from build123d import *

# Parameters (mm, degrees)
SKETCH1_R              = 56.531668112
BOSS_EXTRUDE1_DEPTH    = 5
CUT_EXTRUDE1_START     = -9.696123263
CUT_EXTRUDE1_OUTLINE_R = 56.531668112
CUT_EXTRUDE1_DEPTH     = 5
CUT_EXTRUDE2_DEPTH     = 93.989824492


# Read off the part's stored shape, not the designer's step: Cut-Extrude1
with BuildPart() as part:
    # Sketch1 → Boss-Extrude1 (new body)
    with BuildSketch(Plane(origin=(0, 0, 0), x_dir=(1, 0, 0), z_dir=(0, 1, 0))):
        with Locations(Location((0, 0, 0), (0, 0, 270))):
            Circle(SKETCH1_R)
    extrude(amount=BOSS_EXTRUDE1_DEPTH)

    # Cut-Extrude1 outline → Cut-Extrude1 (cut)
    with BuildSketch(Plane(origin=(0.053951493, 9.696123263, -2.690451675), x_dir=(0, 0, 1), z_dir=(0, 1, 0)).offset(CUT_EXTRUDE1_START)):
        with Locations((2.690451675, -0.053951493)):
            Circle(CUT_EXTRUDE1_OUTLINE_R)
        with BuildLine():
            ThreePointArc((-0.274694701, 5.590628471), (0.097098839, 5.770814345), (0.479781475, 5.926542907))
            ThreePointArc((0.479781475, 5.926542907), (0.311357577, 7.137787092), (0.620358822, 8.321001915))
            ThreePointArc((0.620358822, 8.321001915), (0.896797518, 8.384527858), (1.175175163, 8.438931768))
            ThreePointArc((1.175175163, 8.438931768), (1.938718671, 7.48369337), (2.277513178, 6.308662576))
            ThreePointArc((2.277513178, 6.308662576), (2.690451674, 6.322048507), (3.103390171, 6.308662576))
            ThreePointArc((3.103390171, 6.308662576), (3.442184678, 7.483693371), (4.205728187, 8.438931768))
            ThreePointArc((4.205728187, 8.438931768), (4.484105832, 8.384527858), (4.760544528, 8.321001915))
            ThreePointArc((4.760544528, 8.321001915), (5.069545773, 7.137787092), (4.901121875, 5.926542907))
            ThreePointArc((4.901121875, 5.926542907), (5.283804511, 5.770814345), (5.65559805, 5.590628471))
            ThreePointArc((5.65559805, 5.590628471), (6.443030314, 6.526272375), (7.529092477, 7.088364951))
            ThreePointArc((7.529092477, 7.088364951), (7.761275046, 6.925438117), (7.987976033, 6.754966533))
            ThreePointArc((7.987976033, 6.754966533), (7.789005891, 5.548363877), (7.142485611, 4.510341424))
            ThreePointArc((7.142485611, 4.510341424), (7.428743082, 4.212425253), (7.695105184, 3.89659521))
            ThreePointArc((7.695105184, 3.89659521), (8.795021012, 4.431070894), (10.015811815, 4.502826734))
            ThreePointArc((10.015811815, 4.502826734), (10.161652833, 4.259548507), (10.299417449, 4.011607367))
            ThreePointArc((10.299417449, 4.011607367), (9.626879667, 2.990249439), (8.614052233, 2.304932231))
            ThreePointArc((8.614052233, 2.304932231), (8.754388023, 1.916340863), (8.869262259, 1.519476535))
            ThreePointArc((8.869262259, 1.519476535), (10.091476213, 1.560368296), (11.235909836, 1.129380165))
            ThreePointArc((11.235909836, 1.129380165), (11.270192066, 0.84781556), (11.295199558, 0.56527614))
            ThreePointArc((11.295199558, 0.56527614), (10.265382027, -0.094234996), (9.061374505, -0.308349388))
            ThreePointArc((9.061374505, -0.308349388), (9.03152328, -0.720424975), (8.975046852, -1.12970214))
            ThreePointArc((8.975046852, -1.12970214), (10.108227036, -1.589464859), (10.978420508, -2.448675198))
            ThreePointArc((10.978420508, -2.448675198), (10.895216241, -2.719841103), (10.803142587, -2.98812517))
            ThreePointArc((10.803142587, -2.98812517), (9.594110114, -3.171754047), (8.407106342, -2.8776433))
            ThreePointArc((8.407106342, -2.8776433), (8.212229649, -3.241951493), (7.994167845, -3.592873756))
            ThreePointArc((7.994167845, -3.592873756), (8.84237711, -4.473793803), (9.287866075, -5.612661077))
            ThreePointArc((9.287866075, -5.612661077), (9.101562084, -5.826541234), (8.908327655, -6.034181196))
            ThreePointArc((8.908327655, -6.034181196), (7.729132938, -5.710176712), (6.764376652, -4.958695246))
            ThreePointArc((6.764376652, -4.958695246), (6.438170443, -5.212243849), (6.09622813, -5.444133562))
            ThreePointArc((6.09622813, -5.444133562), (6.512803388, -6.593891859), (6.456558756, -7.81549557))
            ThreePointArc((6.456558756, -7.81549557), (6.199368695, -7.935108156), (5.938385479, -8.046201177))
            ThreePointArc((5.938385479, -8.046201177), (4.992921997, -7.270586652), (4.417228324, -6.191672439))
            ThreePointArc((4.417228324, -6.191672439), (4.016096616, -6.290620595), (3.609398725, -6.363381921))
            ThreePointArc((3.609398725, -6.363381921), (3.52231033, -7.583174812), (2.974057309, -8.67628858))
            ThreePointArc((2.974057309, -8.67628858), (2.690451675, -8.680951493), (2.406846041, -8.67628858))
            ThreePointArc((2.406846041, -8.67628858), (1.85859302, -7.583174812), (1.771504625, -6.363381921))
            ThreePointArc((1.771504625, -6.363381921), (1.364806734, -6.290620595), (0.963675026, -6.191672439))
            ThreePointArc((0.963675026, -6.191672439), (0.387981353, -7.270586652), (-0.557482129, -8.046201177))
            ThreePointArc((-0.557482129, -8.046201177), (-0.818465345, -7.935108156), (-1.075655406, -7.81549557))
            ThreePointArc((-1.075655406, -7.81549557), (-1.131900038, -6.593891859), (-0.71532478, -5.444133562))
            ThreePointArc((-0.71532478, -5.444133562), (-1.057267094, -5.212243849), (-1.383473303, -4.958695246))
            ThreePointArc((-1.383473303, -4.958695246), (-2.348229589, -5.710176712), (-3.527424305, -6.034181196))
            ThreePointArc((-3.527424305, -6.034181196), (-3.720658735, -5.826541234), (-3.906962725, -5.612661077))
            ThreePointArc((-3.906962725, -5.612661077), (-3.46147376, -4.473793803), (-2.613264496, -3.592873756))
            ThreePointArc((-2.613264496, -3.592873756), (-2.8313263, -3.241951493), (-3.026202992, -2.8776433))
            ThreePointArc((-3.026202992, -2.8776433), (-4.213206764, -3.171754047), (-5.422239237, -2.98812517))
            ThreePointArc((-5.422239237, -2.98812517), (-5.514312891, -2.719841103), (-5.597517158, -2.448675198))
            ThreePointArc((-5.597517158, -2.448675198), (-4.727323686, -1.589464859), (-3.594143503, -1.12970214))
            ThreePointArc((-3.594143503, -1.12970214), (-3.65061993, -0.720424975), (-3.680471156, -0.308349388))
            ThreePointArc((-3.680471156, -0.308349388), (-4.884478678, -0.094234996), (-5.914296209, 0.56527614))
            ThreePointArc((-5.914296209, 0.56527614), (-5.889288716, 0.84781556), (-5.855006486, 1.129380165))
            ThreePointArc((-5.855006486, 1.129380165), (-4.710572864, 1.560368296), (-3.48835891, 1.519476535))
            ThreePointArc((-3.48835891, 1.519476535), (-3.373484673, 1.916340863), (-3.233148884, 2.304932231))
            ThreePointArc((-3.233148884, 2.304932231), (-4.245976317, 2.990249439), (-4.9185141, 4.011607367))
            ThreePointArc((-4.9185141, 4.011607367), (-4.780749484, 4.259548507), (-4.634908466, 4.502826734))
            ThreePointArc((-4.634908466, 4.502826734), (-3.414117662, 4.431070894), (-2.314201834, 3.89659521))
            ThreePointArc((-2.314201834, 3.89659521), (-2.047839732, 4.212425253), (-1.761582261, 4.510341424))
            ThreePointArc((-1.761582261, 4.510341424), (-2.408102542, 5.548363877), (-2.607072683, 6.754966533))
            ThreePointArc((-2.607072683, 6.754966533), (-2.380371697, 6.925438117), (-2.148189128, 7.088364951))
            ThreePointArc((-2.148189128, 7.088364951), (-1.062126965, 6.526272376), (-0.274694701, 5.590628471))
        make_face(mode=Mode.SUBTRACT)
    extrude(amount=CUT_EXTRUDE1_DEPTH, mode=Mode.SUBTRACT)

    # Sketch4 → Cut-Extrude2 (cut, through all)
    with BuildSketch(Plane(origin=(64.693992366, 5.1354, -48.358110231), x_dir=(1, 0, 0), z_dir=(0, 1, 0))):
        with BuildLine():
            Line((-64.693992366, -49.758110231), (-63.380949475, -47.872395945))
            ThreePointArc((-63.380949475, -47.872395945), (-65.842904895, -47.558110231), (-64.693992366, -49.758110231))
        make_face()
    extrude(amount=-CUT_EXTRUDE2_DEPTH, mode=Mode.SUBTRACT)


solid = part.part
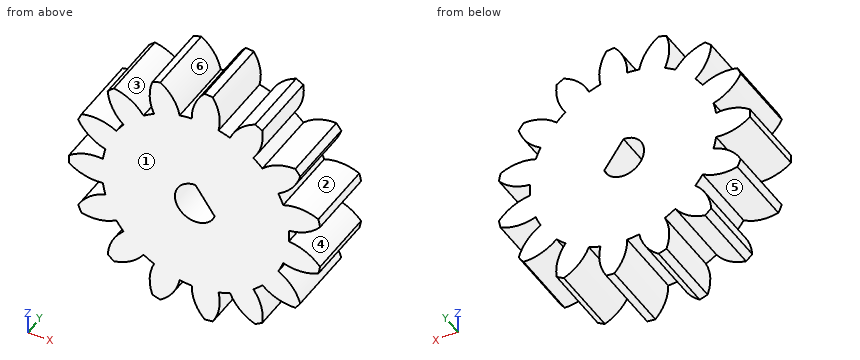
CAD build for the part. Positions are in the model's coordinates, mm. Face numbers are marked on the shaded views. A direction names the side the tool comes from. Give positions to 0.01 mm unless a question says otherwise; leave off trailing zeros. Write each loop counter-clockwise with the first axis right and the second up, starting at its lowest first coordinate (ties: lowest second). Pieces come first, ordered by that corner, then holes. Notation, with made-up numbers: M -10.75,10.5 L 11.25,10.5 A19 cw 11.25,45.5 Z; hole C 32.5,85.25 d10. An arc over 180 degrees is marked long. Put each result on its own line as item: value. Start each with the question number.
(1) Flat gauge pin, fed straight in: pin 1 Ø1.5 at (x, y) = (-7, 1.5) entering from -Z. Where does the tip first touch, or does it go through?
(2) Band-saw the part on B-B, the plane x = 3. Write the cut outline in (y, z).
(3) Probe L1, parallel to X at y = 1.7, z = -7.5; L2, parallel to X at y = 2.55, z = 6.75; L3, parallel to X at y = 3.5, z = 0. List the from-to ranges inside material, lowest first.
(4) Which spindle directions (+Z, -Z, +X, -X, +Y, -Y) get a long thin tool onto all of the face, cutting with end or side? Do the marked faces 4, 5 and 6. Say none if no direction does.
(5) Mould opens along Z. For the marked faces 1, 2 and 3 say: +Z half, -Z half, draft (parallel to the pull), parting line (faces both ways), or undercut.
(6) Band-saw the part on A-A, the plane z = 0. Write the cut outline in (x, y), and give its area (3 significant figures).
Response values:
1. pin 1: stops at z = -3.86
2. outline: M 0,-6.89 L 5,-6.89 L 5,6.89 L 0,6.89 Z
3. L1: x = -3.09 to -1.59, -0.07 to 1.6, 3.83 to 4.26
3. L2: x = -3.11 to -1.2, -0.24 to 1.65, 2.87 to 4.58
3. L3: x = -8.63 to -1.4, 0.97 to 6.38
4. face 4: +X, +Y, -Y
4. face 5: +Y, -Y
4. face 6: +Z, +Y, -Y
5. face 1: draft
5. face 2: undercut
5. face 3: +Z half
6. outline: M -8.63,0 L -1.4,0 L -1.4,5 L -8.63,5 Z; M 0.97,0 L 6.38,0 L 6.38,5 L 0.97,5 Z
6. area: 63.1 mm2
